Can you work these out from the model? Positions are in its coordinate system, mm. A direction names the side the tool comes from. Round coordinates to 2 decimals unless told otherwise and drop trailing zeros. Write each loop counter-clockwise with the first axis right and the second up, starting at its lowest first coordinate (ties: lowest second). Pieces come first, ordered by that corner, then holes. Notation, with made-up numbers: M 28,-20.75 L 46,-20.75 A22 cw 46,-1.75 Z; hole C 33,86 d2. An arc over 180 degrees is marked long. Answer as a JSON object with one key per item and string values. Group by question number.
1) Please list where these lines run through material, in increasing order: L1, parallel to Y at x = 39, z = -10; L2, parallel to Z at x = 67, y = 13.5 (3 decimals); L3, parallel to Z at x = 37, y = 12. Write a range as [from, to].
2) Suppose I cut it at D-D, the plane x = 18. Write out the boundary of the cut face in (y, z) (3 decimals).
3) On a 3-axis mill with a long thin cutter (end or side, diameter ignored), from which of +Z, -Z, +X, -X, +Y, -Y can I reach the whole of each face in a straight line? I mean faces 4 (the cylindrical face through (57.08, 27.05, -4.83)), 5 (the flat face through (39, 25, -9.525)), 6 (the flat face through (38, 14.263, -19)). Say none if no direction works.
4) I'm going to push flat-ended pins straight in: pin 1 Ø6 at (x, y) = (60.32, 26.03) entering from +Z; pin 2 Ø5 at (x, y) = (64.5, 21) entering from +Z; pin 3 Ø3 at (x, y) = (24, 35) entering from -Z. Where does each tip first touch, or does it pass through?
5) Suppose I cut it at A-A, the plane x = 38.1. Write out the boundary of the cut face in (y, z) (3 decimals), and give its area (3 significant figures).
6) If we mould it in two halves opening along Z, with no side actions, what happens to faces 1 (the flat face through (24.845, 11.526, -22.725)), 2 (the flat face through (5.08, 24, -5)), 3 (the cylindrical face through (41.336, 37.727, -27.505))? For each: +Z half, -Z half, draft (parallel to the pull), parting line (faces both ways), or undercut.
7) Suppose I cut it at B-B, the plane y = 12. Write out the boundary of the cut face in (x, z) (3 decimals).
8) Suppose I cut it at C-C, the plane z = -20.5. Write out the boundary of the cut face in (x, y), and give its area (3 significant figures).
from build123d import *

# Parameters (mm, degrees)
BOSS_EXTRUDE1_DEPTH = 76.2
SKETCH2_R           = 3.4
CUT_EXTRUDE1_DEPTH  = 9.525
CUT_EXTRUDE2_REACH  = 93.635
SKETCH3_R           = 3.2639
SKETCH4_W           = 5.08
SKETCH4_H           = 31.75
CUT_EXTRUDE3_DEPTH  = 9.525


with BuildPart() as part:
    # Sketch1 → Boss-Extrude1 (new body)
    with BuildSketch(Plane(origin=(0, 0, 0), x_dir=(0, 0, -1), z_dir=(1, 0, 0))):
        Polygon((0, 8.712610854), (0, 40.462610854), (39.779713659, 40.462610854), (39.779713659, 34.912710854), (9.525, 34.912710854), (9.525, 14.262510854), (39.779713659, 14.262510854), (39.779713659, 8.712610854), align=None)
    extrude(amount=BOSS_EXTRUDE1_DEPTH)

    # Sketch2 → Cut-Extrude1 (cut)
    with BuildSketch(Plane(origin=(0, 0, -9.525), x_dir=(-1, 0, 0), z_dir=(0, 0, -1))):
        with Locations((-60.325, 26.02985118)):
            Circle(SKETCH2_R)
        with Locations((-15.875, 26.02985118)):
            Circle(SKETCH2_R)
    extrude(amount=-CUT_EXTRUDE1_DEPTH, mode=Mode.SUBTRACT)

    # Cut-Extrude2: up to this face of the body (flat: up to its plane)
    cut_extrude2_end = Plane(part.part.faces().sort_by_distance((38.1, 8.712610854, -19.889856829))[0])
    # Sketch3 → Cut-Extrude2 (cut, up to the picked face)
    with BuildSketch(Plane(origin=(0, 40.462610854, 0), x_dir=(1, 0, 0), z_dir=(0, 1, 0)), mode=Mode.PRIVATE) as cut_extrude2_sk1:
        with Locations(Location((38.1, 27.079713659, 0), (0, 0, 270))):
            Circle(SKETCH3_R)
    cut_extrude2_tool1 = split(extrude(cut_extrude2_sk1.sketch, amount=-CUT_EXTRUDE2_REACH, mode=Mode.PRIVATE), bisect_by=cut_extrude2_end, keep=Keep.BOTH, mode=Mode.PRIVATE)
    # Sketch3 → Cut-Extrude2 (cut, up to the picked face)
    with BuildSketch(Plane(origin=(0, 40.462610854, 0), x_dir=(1, 0, 0), z_dir=(0, 1, 0)), mode=Mode.PRIVATE) as cut_extrude2_sk2:
        Polygon((30.48, 35.56), (19.05, 9.525), (0, 9.525), (0, 39.779713659), (76.2, 39.779713659), (76.2, 9.525), (57.15, 9.525), (45.72, 35.56), align=None)
    cut_extrude2_tool2 = split(extrude(cut_extrude2_sk2.sketch, amount=-CUT_EXTRUDE2_REACH, mode=Mode.PRIVATE), bisect_by=cut_extrude2_end, keep=Keep.BOTH, mode=Mode.PRIVATE)
    add(cut_extrude2_tool1.solids().sort_by(Axis((38.1, 40.462611, -27.079714), (0, -1, 0)))[0], mode=Mode.SUBTRACT)
    add(cut_extrude2_tool2.solids().sort_by(Axis((24.014295, 40.462611, -22.872078), (0, -1, 0)))[0], mode=Mode.SUBTRACT)

    # Sketch4 → Cut-Extrude3 (cut)
    with BuildSketch(Plane(origin=(0, 0, -9.525), x_dir=(-1, 0, 0), z_dir=(0, 0, -1))):
        with Locations((-2.54, 24.587610854)):
            Rectangle(SKETCH4_W, SKETCH4_H)
        with Locations((-73.66, 24.587610854)):
            Rectangle(SKETCH4_W, SKETCH4_H)
    extrude(amount=-CUT_EXTRUDE3_DEPTH, mode=Mode.SUBTRACT)


solid = part.part
Results:
{
 "1": {"L1": "[8.71, 14.26], [34.91, 40.46]", "L2": "[-9.525, 0]", "L3": "[-35.56, -30.15], [-24.01, 0]"},
 "2": {"outline": "M 8.713,-9.525 L 23.376,-9.525 L 23.376,0 L 8.713,0 Z; M 28.684,-9.525 L 40.463,-9.525 L 40.463,0 L 28.684,0 Z"},
 "3": {"face 4": "+Z, -Z", "face 5": "-Z", "face 6": "-Z, +X, -X"},
 "4": {"pin 1": "through", "pin 2": "z = 0", "pin 3": "z = -24.22"},
 "5": {"outline": "M 8.713,-35.56 L 14.263,-35.56 L 14.263,-30.344 L 8.713,-30.344 Z; M 8.713,-23.816 L 14.263,-23.816 L 14.263,-9.525 L 34.913,-9.525 L 34.913,-23.816 L 40.463,-23.816 L 40.463,0 L 8.713,0 Z; M 34.913,-35.56 L 40.463,-35.56 L 40.463,-30.344 L 34.913,-30.344 Z", "area": "519 mm^2"},
 "6": {"face 1": "-Z half", "face 2": "draft", "face 3": "undercut"},
 "7": {"outline": "M 5.08,-9.525 L 19.05,-9.525 L 30.48,-35.56 L 45.72,-35.56 L 57.15,-9.525 L 71.12,-9.525 L 71.12,0 L 5.08,0 Z; hole C 38.1,-27.08 d6.528"},
 "8": {"outline": "M 23.87,8.71 L 52.33,8.71 L 52.33,14.26 L 23.87,14.26 Z; M 23.87,34.91 L 52.33,34.91 L 52.33,40.46 L 23.87,40.46 Z", "area": "316 mm^2"}
}
